Can you work these out from the model? Positions are in its coordinate system, mm. A direction names the side the tool comes from. Round coordinates to 2 decimals unless told otherwise and drop trailing zeros. Loops run counter-clockwise (first coordinate to the right, second up) from the corner with the lowest first, then second, coordinate; pieces in that order, holes last.
(1) I want a section at A-A on z = -7.5. Write out the boundary of the cut face in (x, y).
(2) Which directions (+Z, -Z, +X, -X, +Y, -Y) give clear straight access to the entire face, cutting with the end or side of a thin tool? Please do faces 5 (the face through (-14, -3, -27.216)), 6 (the face through (-50.8, -3, 7)).
(3) If I drill on line 1 along Z through (x, y) = (-39, -5); line 2 along X through (y, z) = (-3.5, -17.5); line 3 along Z through (x, y) = (-16, -4.75), over which ranges is the centre line in solid material (lowest first)?
(4) Thinking about a two-plate mould opening in Z: for faces 1 (the face through (-38, -3, 48.984)), 2 (the face through (-49.93, -3.13, -39)), 3 (the face through (-37.61, -3.13, 37.59)), 4 (the face through (-37, -6.35, 5)), which applies, released by +Z, released by -Z, zero draft, split by the parting line, or undercut?
(5) I want a section at B-B on x = -19.5. Write out the boundary of the cut face in (y, z), plus the area to 3 significant figures.
(6) Will these pins go through, and if not, where does the flat tip stop? pin 1 Ø1.9 at (x, y) = (-14, -2.5) entering from +Z; pin 2 Ø3 at (y, z) = (-3.5, -6) entering from +X.
from build123d import *

# Parameters (mm, degrees)
F0_W     = 25.4
F0_H     = 76.2
F0_R     = 2.3495
F1_DEPTH = 6.35


with BuildPart() as f1:
    # F0 (on Front) → F1 (new body)
    with BuildSketch(Plane.XZ):
        with Locations((-38.1, 10.883943)):
            Rectangle(F0_W, F0_H)
        with Locations((-38.690675, 39.674234)):
            Circle(F0_R, mode=Mode.SUBTRACT)
        with BuildLine():
            Line((-25.4, -27.216057), (-50.8, -27.216057))
            Line((-50.8, -27.216057), (-50.8, -36.868057))
            ThreePointArc((-50.8, -36.868057), (-49.907261, -39.023318), (-47.752, -39.916057))
            Line((-47.752, -39.916057), (-3.048, -39.916057))
            ThreePointArc((-3.048, -39.916057), (-0.892739, -39.023318), (0, -36.868057))
            Line((0, -36.868057), (0, -36.396314))
            add(Edge.make_bspline(
                [(0, -30.599461), (-16.314539, -28.600201), (-16.314539, -33.497887), (-16.314539, -38.395574), (0, -36.396314)],
                knots=[1.150309, 1.150309, 1.150309, 3.141593, 3.141593, 5.132876, 5.132876, 5.132876], degree=2, weights=[1, 0.543965, 1, 0.543965, 1]))
            Line((0, -30.599461), (0, -30.264057))
            ThreePointArc((0, -30.264057), (-0.892739, -28.108795), (-3.048, -27.216057))
            Line((-3.048, -27.216057), (-25.4, -27.216057))
        make_face()
    extrude(amount=F1_DEPTH)


solid = f1.part
Filled sheet:
1. outline: (-50.8, -6.35) - (-25.4, -6.35) - (-25.4, 0) - (-50.8, 0) - close
2. face 5: +Z, +X, +Y, -Y
2. face 6: +Z, -Z, -X, +Y, -Y
3. line 1: z = -39.92 to 37.35, 42 to 48.98
3. line 2: x = -50.8 to -25.4
3. line 3: z = -39.92 to -34.23, -32.76 to -27.22
4. face 1: released by +Z
4. face 2: released by -Z
4. face 3: undercut
4. face 4: zero draft
5. outline: (-6.35, -39.92) - (0, -39.92) - (0, -27.22) - (-6.35, -27.22) - close
5. area: 80.6 mm2
6. pin 1: stops at z = -27.22
6. pin 2: stops at x = -25.4
